Model file for the job. Use its own axes, mm. A direction names the side the tool comes from. Coordinates: 2 decimals unless noted, no trailing zeros. Order: outer loops, then holes, each group sorted by start corner. A loop starts at its lowest first (then second) coordinate and runs counter-clockwise, first axis right, second up. Notation, with made-up numbers: (-10.75, 35) -> (23.25, 35) arc R19 cw to (23.25, 40) -> close; hole circle Ø5 at (3.5, 63.5). An arc over 180 degrees is marked (long way). Return JSON: item names as keys, results as strings. Group by question number.
1) Cut at A-A (y = 4). Write the cut outline in (x, z) (1 decimal), and give its area (3 significant figures).
2) Probe line 1 (Z direction, x = 39, y = -14) (3 decimals); line 2 (X direction, y = 26, z = -2.75); line 3 (X direction, y = -2.5, z = -1.25). List the from-to ranges inside material, lowest first.
3) Which spindle directions (+Z, -Z, +X, -X, +Y, -Y) get a long thin tool onto all of the face, cutting with end or side? Do faces 1 (the flat face through (-38, -26, -3.969)), 2 (the cylindrical face through (-38.982, 20.685, -1.957)), 3 (the flat face through (42, 5, 8.509)), 4 (the flat face through (-30.321, 0, -2)). Say none if no direction does.
4) Pull direction Y, two halves, no side cores. Call faces 5 (the flat face through (-35, -3, 0)), 6 (the flat face through (-1, -34.925, 11)), 7 (the flat face through (46.99, 0, 8)): +Y half, -Y half, draft (parallel to the pull), parting line (faces both ways), or undercut.
5) Cut at B-B (x = -26). Write the cut outline in (y, z) (3 decimals).
6) Flat gauge pins, fed straight in: pin 1 (5.5 mm diameter, centred on x = -39, y = -28.5, fed in from -Z); pin 2 (0.6 mm diameter, centred on x = 42.5, y = 0, fed in from -Z); pin 3 (1.7 mm diameter, centred on x = 41.5, z = 17, fed in from -Y). Where does each tip first touch, or does it go through?
from build123d import *

# Parameters (mm, degrees)
F0_W      = 93.98
F0_H      = 69.85
F1_DEPTH  = 22.225
F2_W      = 10.31875
F2_H      = 15.875
F3_DEPTH  = 4.7625
F4_R      = 5.08
F5_R      = 5.55625
F6_DEPTH  = 3.96875
F8_R      = 7.62
F9_W      = 7.874
F9_H      = 1.524
F9_W_2    = 1.905
F9_H_2    = 6.604
F10_DEPTH = 10.668
F11_DEPTH = 10.668
F9_R      = 3.048
F12_DEPTH = 10.668
F13_R     = 0.635
F14_DEPTH = 10.668
F15_R     = 0.6096
F7_R      = 3.96875
F16_DEPTH = 4.7625


with BuildPart() as f1:
    # F0 (on Top) → F1 (new body)
    with BuildSketch(Plane.XY):
        Rectangle(F0_W, F0_H)
    extrude(amount=F1_DEPTH)

    # F2 (on face) → F3 (join)
    with BuildSketch(Plane(origin=(0, 0, 0), x_dir=(1, 0, 0), z_dir=(0, 0, -1))):
        with Locations((-35.480625, 0)):
            Rectangle(F2_W, F2_H)
        with Locations((35.480625, 0)):
            Rectangle(F2_W, F2_H)
    extrude(amount=F3_DEPTH)

    # F4
    f4_edges = [f1.edges().sort_by_distance(p)[0] for p in [
        (-30.32125, -7.9375, -2.38125),
        (-40.64, -7.9375, -2.38125),
        (30.32125, -7.9375, -2.38125),
        (40.64, -7.9375, -2.38125),
        (40.64, 7.9375, -2.38125),
        (30.32125, 7.9375, -2.38125),
        (-30.32125, 7.9375, -2.38125),
        (-40.64, 7.9375, -2.38125),
    ]]
    fillet(f4_edges, radius=F4_R)

    # F5 (on face) → F6 (join)
    with BuildSketch(Plane(origin=(0, 0, 0), x_dir=(1, 0, 0), z_dir=(0, 0, -1))):
        with Locations((38.25875, 26.19375)):
            Circle(F5_R)
        with Locations((-38.25875, -26.19375)):
            Circle(F5_R)
        with Locations((38.25875, -26.19375)):
            Circle(F5_R)
        with Locations((-38.25875, 26.19375)):
            Circle(F5_R)
    extrude(amount=F6_DEPTH)

    # F8
    f8_edges = [f1.edges().sort_by_distance(p)[0] for p in [
        (-46.99, -34.925, 11.1125),
        (46.99, -34.925, 11.1125),
        (46.99, 34.925, 11.1125),
        (-46.99, 34.925, 11.1125),
    ]]
    fillet(f8_edges, radius=F8_R)

    # F9 (on face) → F10 (cut)
    with BuildSketch(Plane.YZ.offset(46.99)):
        with Locations((-10.643445003, 17.399)):
            Rectangle(F9_W, F9_H)
        with Locations((-5.753945003, 13.335)):
            Rectangle(F9_W_2, F9_H_2)
        with Locations((-10.643445003, 13.335)):
            Rectangle(F9_W, F9_H_2)
        with Locations((-15.532945003, 13.335)):
            Rectangle(F9_W_2, F9_H_2)
        with Locations((-10.643445003, 9.271)):
            Rectangle(F9_W, F9_H)
    extrude(amount=-F10_DEPTH, mode=Mode.SUBTRACT)

    # F9 (on face) → F11 (cut)
    with BuildSketch(Plane.YZ.offset(46.99)):
        with Locations((-0.292945003, 13.335)):
            Rectangle(F9_W_2, F9_H_2)
        with Locations((4.596554997, 17.399)):
            Rectangle(F9_W, F9_H)
        with Locations((4.596554997, 9.271)):
            Rectangle(F9_W, F9_H)
        with Locations((4.596554997, 13.335)):
            Rectangle(F9_W, F9_H_2)
        with Locations((9.486054997, 13.335)):
            Rectangle(F9_W_2, F9_H_2)
    extrude(amount=-F11_DEPTH, mode=Mode.SUBTRACT)

    # F9 (on face) → F12 (cut)
    with BuildSketch(Plane.YZ.offset(46.99)):
        with Locations((-23.368, 15.4551044106)):
            Circle(F9_R)
    extrude(amount=-F12_DEPTH, mode=Mode.SUBTRACT)

    # F13 (on face) → F14 (join)
    with BuildSketch(Plane.YZ.offset(36.322)):
        with Locations((-23.368, 15.4551044106)):
            Circle(F13_R)
    extrude(amount=F14_DEPTH)

    # F15
    f15_edges = [f1.edges().sort_by_distance(p)[0] for p in [
        (46.99, -24.003, 15.455104),
    ]]
    fillet(f15_edges, radius=F15_R)

    # F7 (on face) → F16 (cut)
    with BuildSketch(Plane(origin=(0, 0, -4.7625), x_dir=(1, 0, 0), z_dir=(0, 0, -1))):
        with Locations((-35.40125, 2.8575)):
            Circle(F7_R)
        with Locations((35.40125, 2.8575)):
            Circle(F7_R)
    extrude(amount=-F16_DEPTH, mode=Mode.SUBTRACT)


solid = f1.part
Answers below:
{
 "1": {"outline": "(-47, 0) -> (-40.5, 0) -> (-40.5, -4.8) -> (-30.5, -4.8) -> (-30.5, 0) -> (30.5, 0) -> (30.5, -4.8) -> (40.5, -4.8) -> (40.5, 0) -> (47, 0) -> (47, 8.5) -> (36.3, 8.5) -> (36.3, 18.2) -> (47, 18.2) -> (47, 22.2) -> (-47, 22.2) -> close", "area": "2,080 mm^2"},
 "2": {"line 1": "z = 0 to 8.509, 18.161 to 22.225", "line 2": "x = -43.81 to -32.71, 32.71 to 43.81", "line 3": "x = -40.64 to -39.35, -31.45 to -30.32, 30.32 to 31.45, 39.35 to 40.64"},
 "3": {"face 1": "-Z, +X, -X, -Y", "face 2": "-Z", "face 3": "+X", "face 4": "-Z, +Y, -Y"},
 "4": {"face 5": "undercut", "face 6": "-Y half", "face 7": "draft"},
 "5": {"outline": "(-34.925, 0) -> (34.925, 0) -> (34.925, 22.225) -> (-34.925, 22.225) -> close"},
 "6": {"pin 1": "stops at z = -3.97", "pin 2": "stops at z = 0", "pin 3": "stops at y = -34.82"}
}
